from build123d import *

# Parameters (mm, degrees)
F0_W     = 445
F0_H     = 370
F1_DEPTH = 60
F2_W     = 30
F2_H     = 50
F3_DEPTH = 240
F4_W     = 505
F4_H     = 240
F5_DEPTH = 10
F6_W     = 40
F6_H     = 430
F7_DEPTH = 8


with BuildPart() as f1:
    # F0 (on Front) → F1 (new body)
    with BuildSketch(Plane.XZ):
        Polygon((505, 750), (0, 750), (0, 0), (30, 0), (30, 320), (475, 320), (475, 0), (505, 0), align=None)
        with Locations((252.5, 535)):
            Rectangle(F0_W, F0_H, mode=Mode.SUBTRACT)
    extrude(amount=F1_DEPTH)

    # F2 (on face) → F3 (join)
    with BuildSketch(Plane.XZ.offset(60)):
        with Locations((15, 25)):
            Rectangle(F2_W, F2_H)
        with Locations((490, 25)):
            Rectangle(F2_W, F2_H)
    extrude(amount=F3_DEPTH)

    # F4 (on face) → F5 (join)
    with BuildSketch(Plane.XY.offset(50)):
        with Locations((252.5, -180)):
            Rectangle(F4_W, F4_H)
    extrude(amount=F5_DEPTH)

    # F6 (on face) → F7 (join)
    with BuildSketch(Plane(origin=(0, 0, 0), x_dir=(-1, 0, 0), z_dir=(0, 1, 0))):
        with Locations((-252.5, 535)):
            Rectangle(F6_W, F6_H)
    extrude(amount=F7_DEPTH)


solid = f1.part
Read the model definition and answer for the solid it produces. Units are mm, in the model's axes. A direction names the side the tool comes from. Coordinates: 2 decimals unless noted, no trailing zeros. Loops run counter-clockwise (first coordinate to the right, second up) from the corner with the lowest first, then second, coordinate; pieces in that order, holes last.
Q1. The part is cut by section B-B on z = 685. Write down the section's boundary in (x, y), and give its area (3 significant figures).
Q2. The mould has two halves that part along Z. Classify faces 5 (the face through (483, 0, 432)), 6 (the face through (475, -30, 532)), 7 (the face through (490, -148, 0)), 8 (the face through (253, 0, 538)): +Z half, -Z half, draft (parallel to the pull), parting line (faces both ways), or undercut.
Q3. Which of the six approach directions +Z, -Z, +X, -X, +Y, -Y give full straight-line access (tool end or side, diameter ignored) to faces 1 (the face through (29.6, 0, 432.3)), 2 (the face through (30, -30, 532)), 3 (the face through (214, -60, 330)), 4 (the face through (256, -26, 320))?
Q4. Consider probe 1 along X at (y, z) = (-49, 99); probe 2 along Z at (x, y) = (273.5, -34.5); probe 3 along Z at (x, y) = (190, -137). Determine where each line is inside the solid, lowest interval first.
Q5. The part is cut by section A-A on x = 251. Write down the section's boundary in (y, z).
Q6. The part is cut by section D-D on x = 407. Write down the section's boundary in (y, z).
Q7. The part is cut by section C-C on z = 214.5. Write down the section's boundary in (x, y), and give its area (3 significant figures).
Q8. Each of these flat-tipped pins is pushed along its axis until it touches: pin 1 Ø10 at (x, y) = (74.5, -223.5) entering from -Z; pin 2 Ø6 at (x, y) = (215, -101) entering from +Z; pin 3 Ø20.5 at (x, y) = (348.5, -39) entering from -Z. Where does it stop, or does it pass through?
Results below:
1. outline: (0, -60) - (30, -60) - (30, 0) - (0, 0) - close; (232.5, 0) - (272.5, 0) - (272.5, 8) - (232.5, 8) - close; (475, -60) - (505, -60) - (505, 0) - (475, 0) - close
1. area: 3,920 mm2
2. face 5: draft
2. face 6: undercut
2. face 7: -Z half
2. face 8: undercut
3. face 1: +Z, -Z, -X, +Y
3. face 2: +Y, -Y
3. face 3: +Z, +X, -X, -Y
3. face 4: -Z, +Y, -Y
4. probe 1: x = 0 to 30, 475 to 505
4. probe 2: z = 320 to 350, 720 to 750
4. probe 3: z = 50 to 60
5. outline: (-300, 50) - (-60, 50) - (-60, 60) - (-300, 60) - close; (-60, 320) - (8, 320) - (8, 750) - (-60, 750) - (-60, 720) - (0, 720) - (0, 350) - (-60, 350) - close
6. outline: (-300, 50) - (-60, 50) - (-60, 60) - (-300, 60) - close; (-60, 320) - (0, 320) - (0, 350) - (-60, 350) - close; (-60, 720) - (0, 720) - (0, 750) - (-60, 750) - close
7. outline: (0, -60) - (30, -60) - (30, 0) - (0, 0) - close; (475, -60) - (505, -60) - (505, 0) - (475, 0) - close
7. area: 3,600 mm2
8. pin 1: stops at z = 50
8. pin 2: stops at z = 60
8. pin 3: stops at z = 320
